from build123d import *

# Parameters (mm, degrees)
F0_W      = 5
F0_H      = 100
F2_W      = 4.3588989435
F2_H      = 9
F3_DEPTH  = 9
F4_R      = 3.25
F5_DEPTH  = 5
F6_R      = 4.49999
F7_W      = 4.3588989435
F7_H      = 9
F8_DEPTH  = 9
F9_R      = 3.25
F10_DEPTH = 5
F11_R     = 4.49999


# Not quite as in the source:
# - a fillet or chamfer is up to 0.001 mm smaller than in the source, because OpenCascade refuses the exact size


with BuildPart() as f1:
    # F0 (on Top) → F1 (revolve)
    with BuildSketch(Plane.XY):
        with Locations((-2.5, 50)):
            Rectangle(F0_W, F0_H)
    revolve(axis=Axis((0, 50, 0), (0, -1, 0)))

    # F2 (on face) → F3 (join)
    with BuildSketch(Plane.XZ):
        Rectangle(F2_W, F2_H)
    extrude(amount=F3_DEPTH)

    # F4 (on face) → F5 (cut)
    with BuildSketch(Plane.YZ.offset(2.1794494718)):
        with Locations((-4.5, 0)):
            Circle(F4_R)
    extrude(amount=-F5_DEPTH, mode=Mode.SUBTRACT)

    # F6 (radius 4.5 in the source; OpenCascade refuses exactly that, so slightly less here)
    f6_edges = [f1.edges().sort_by_distance(p)[0] for p in [
        (0, -9, 4.5),
        (0, -9, -4.5),
    ]]
    fillet(f6_edges, radius=F6_R)

    # F7 (on face) → F8 (join)
    with BuildSketch(Plane(origin=(0, 100, 0), x_dir=(-1, 0, 0), z_dir=(0, 1, 0))):
        Rectangle(F7_W, F7_H)
    extrude(amount=F8_DEPTH)

    # F9 (on face) → F10 (cut)
    with BuildSketch(Plane(origin=(-2.1794494718, 0, 0), x_dir=(0, -1, 0), z_dir=(-1, 0, 0))):
        with Locations((-104.5, 0)):
            Circle(F9_R)
    extrude(amount=-F10_DEPTH, mode=Mode.SUBTRACT)

    # F11 (radius 4.5 in the source; OpenCascade refuses exactly that, so slightly less here)
    f11_edges = [f1.edges().sort_by_distance(p)[0] for p in [
        (0, 109, 4.5),
        (0, 109, -4.5),
    ]]
    fillet(f11_edges, radius=F11_R)


solid = f1.part
For this review, take the finished solid that the model builds, in its own axes (mm). A direction names the side the tool comes from. Round coordinates to 2 decimals unless told otherwise and drop trailing zeros. Order: outer loops, then holes, each group sorted by start corner. A loop starts at its lowest first (then second) coordinate and runs counter-clockwise, first axis right, second up. Notation, with made-up numbers: M 45,23 L 89,23 A24 cw 89,51 Z; hole C -36,77 d2. An arc over 180 degrees is marked long. Use a Markdown table: item, result. Add a question column.
Item 1: Tool access review of faces 4 (the flat face through (0, -2, -4.5)), 5 (the flat face through (0, 102, 4.5)), 6 (the flat face through (3, 100, 0)), 7 (the flat face through (-3, 100, 0)): name each direction out of +Z, -Z, +X, -X, +Y, -Y from which nothing blocks a thin tool from reaching the whole face with its end or side.
Item 2: Mouldability with a two-part tool opening along Y and no side actions: class faces 1 (the cylindrical face through (0.03, -1.4, 0.98)), 2 (the cylindrical face through (0.031, -7.647, -3.217)), 3 (the flat face through (-2.179, 101, 2)) as released by +Y, released by -Y, zero draft, split by the parting line, or undercut.
Item 3: Add section A-A, the plane z = 1.75. Give the boundary of the cut face in (x, y), then the cut area to 3 significant figures.
Item 4: Add section C-C, the plane y = 98. Give the boundary of the cut face in (x, z).
Item 5: To check wall thickness, follow line 1 along Y through (x, z) = (1, 1); line 2 along Z through (x, y) = (-0.7, -4.5); line 3 along Y through (x, z) = (-1.25, 2). State the ranges of each line that lie inside material, in increasing order.
Item 6: Insertion check: pin 1 (5 mm diameter, centred on x = -1, y = -1.5, fed in from -Z); pin 2 (1.5 mm diameter, centred on y = 15.5, z = 3, fed in from -X); pin 3 (2 mm diameter, centred on x = 0.5, y = 103.5, fed in from -Z); pin 4 (1.5 mm diameter, centred on x = 4, y = 59.5, fed in from -Z). Each pin has a flat end and moves straight along its axis. Give the tip position at first contact, or say it passes through.
Item 7: Add section B-B, the plane x = 0. State how many separate pieces and enclosed holes the cut face has, then the cut area to 3 significant figures.
Geometry results:
| question | item | result |
|---|---|---|
| 1 | face 4 | -Z, +X, -X, -Y |
| 1 | face 5 | +Z, +X, -X, +Y |
| 1 | face 6 | +Z, -Z, +X, +Y |
| 1 | face 7 | +Z, -Z, -X, +Y |
| 2 | face 1 | undercut |
| 2 | face 2 | released by -Y |
| 2 | face 3 | zero draft |
| 3 | outline | M -4.68,0 L -2.18,0 L -2.18,-1.76 L 2.18,-1.76 L 2.18,0 L 4.68,0 L 4.68,100 L 2.18,100 L 2.18,101.76 L -2.18,101.76 L -2.18,100 L -4.68,100 Z; M -2.18,-8.65 L 2.18,-8.65 L 2.18,-7.24 L -2.18,-7.24 Z; M -2.18,107.24 L 2.18,107.24 L 2.18,108.65 L -2.18,108.65 Z |
| 3 | area | 964 mm² |
| 4 | outline | C 0,0 d10 |
| 5 | line 1 | y = -8.89 to -7.59, -1.41 to 101.41, 107.59 to 108.89 |
| 5 | line 2 | z = -4.5 to -3.25, 3.25 to 4.5 |
| 5 | line 3 | y = -8.53 to -7.06, -1.94 to 101.94, 107.06 to 108.53 |
| 6 | pin 1 | stops at z = -5 |
| 6 | pin 2 | stops at x = -4.47 |
| 6 | pin 3 | stops at z = -4.5 |
| 6 | pin 4 | stops at z = -3.8 |
| 7 | separate pieces | 1 |
| 7 | enclosed holes | 2 |
| 7 | area | 1,080 mm² |
